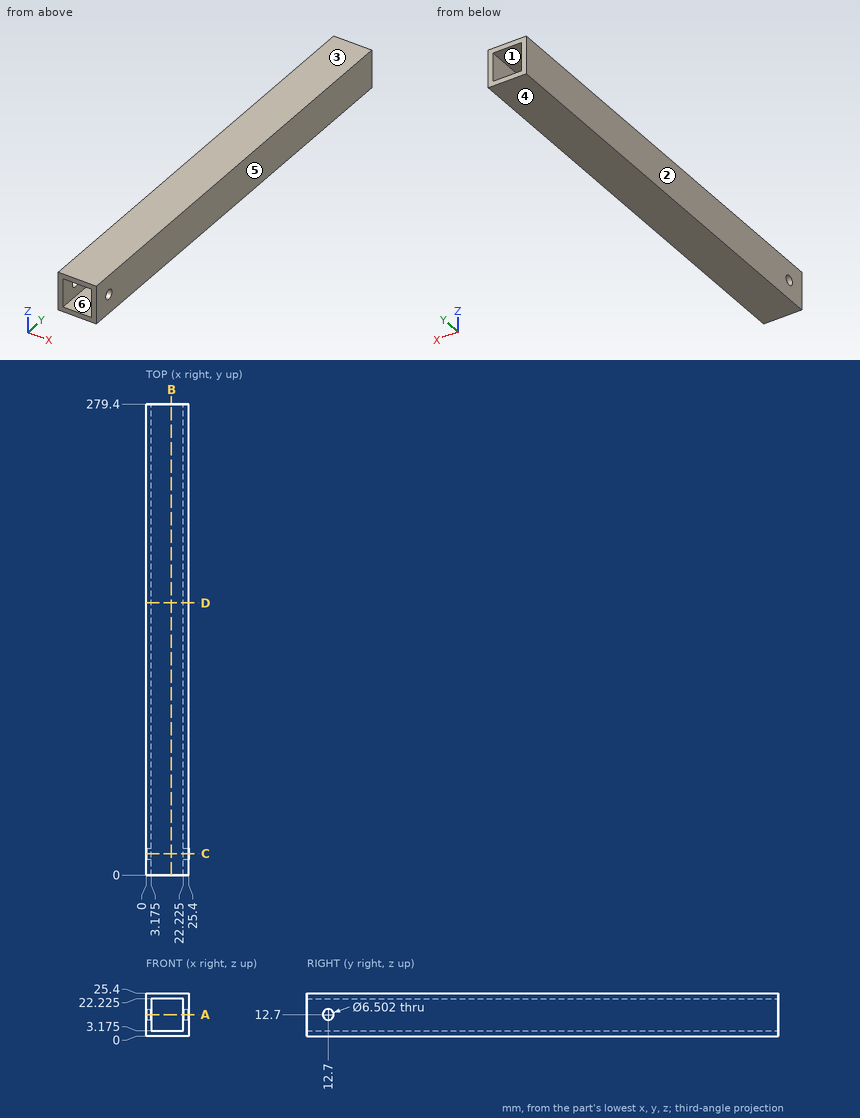
Print and shaded views of the part. All mm, measured from the part's lowest x, y and z. A direction names the side the tool comes from. Round coordinates to 2 decimals unless told otherwise and drop trailing zeros. Write each loop counter-clockwise with the first axis right and the second up, starting at its lowest first coordinate (ties: lowest second). Pieces come first, ordered by that corner, then holes. Notation, with made-up numbers: M 76.5,82 L 112.5,82 A16 cw 112.5,113 Z; hole C 36.5,82 d1. An arc over 180 degrees is marked long. Use a Markdown table: item, result. Add a question column.
1. Slice it at D-D on y = 161.5. Give the cut face in (x, z) (1 decimal).
2. Drill centre lines: probe 1 along Z at (x, y) = (13.75, 184.5) (1 decimal); probe 2 along Y at (x, z) = (24.5, 12.7). Where is each one in solid material? Low to high.
3. 3-axis set-ups, long thin cutter, end or side, ignore diameter. For the marked faces 5 and 6: which of +Z, -Z, +X, -X, +Y, -Y reach the whole face in a straight line?
4. Slice it at B-B on x = 15. Give the cut face in (y, z) (1 decimal).
5. Slice it at A-A on z = 12.7. Give the cut face in (x, y) (1 decimal).
6. Slice it at C-C on y = 12.7. Give the cut face in (x, z) (1 decimal).
7. Pull direction Z, two halves, no side cores. Call the marked faces 1, 2, 3 and 4: released by +Z, released by -Z, zero draft, split by the parting line, or undercut.
Reply:
| question | item | result |
|---|---|---|
| 1 | outline | M 0,0 L 25.4,0 L 25.4,25.4 L 0,25.4 Z; hole M 3.2,3.2 L 22.2,3.2 L 22.2,22.2 L 3.2,22.2 Z |
| 2 | probe 1 | z = 0 to 3.2, 22.2 to 25.4 |
| 2 | probe 2 | y = 0 to 9.45, 15.95 to 279.4 |
| 3 | face 5 | +Z, -Z, +X, +Y, -Y |
| 3 | face 6 | +Y, -Y |
| 4 | outline | M 0,0 L 279.4,0 L 279.4,3.2 L 0,3.2 Z; M 0,22.2 L 279.4,22.2 L 279.4,25.4 L 0,25.4 Z |
| 5 | outline | M 0,0 L 3.2,0 L 3.2,9.4 L 0,9.4 Z; M 0,16 L 3.2,16 L 3.2,279.4 L 0,279.4 Z; M 22.2,0 L 25.4,0 L 25.4,9.4 L 22.2,9.4 Z; M 22.2,16 L 25.4,16 L 25.4,279.4 L 22.2,279.4 Z |
| 6 | outline | M 0,0 L 25.4,0 L 25.4,9.4 L 22.2,9.4 L 22.2,3.2 L 3.2,3.2 L 3.2,9.4 L 0,9.4 Z; M 0,16 L 3.2,16 L 3.2,22.2 L 22.2,22.2 L 22.2,16 L 25.4,16 L 25.4,25.4 L 0,25.4 Z |
| 7 | face 1 | undercut |
| 7 | face 2 | zero draft |
| 7 | face 3 | released by +Z |
| 7 | face 4 | released by -Z |
